Design review of the part built by this model. Coordinates are the model's own, in mm. Face numbers are marked on the shaded views. Round coordinates to 2 decimals unless told otherwise and drop trailing zeros. Write each loop counter-clockwise with the first axis right and the second up, starting at its lowest first coordinate (ties: lowest second). Pieces come first, ordered by that corner, then holes. Notation, with made-up numbers: M -7,-6 L 49,-6 A18 ccw 49,10 Z; hole C 31.5,2 d10. An arc over 180 degrees is marked long. One line per question, with ' | ' between items. Start each with the question number.
Item 1: Insertion check: pin 1 Ø1.5 at (x, z) = (4.5, 2.5) entering from -Y; pin 2 Ø1 at (y, z) = (9, -3.5) entering from -X; pin 3 Ø4 at (x, y) = (-4, 5) entering from -Z; pin 4 Ø5 at (y, z) = (9, -3.5) entering from +X. Each pin has a flat end and moves straight along its axis. Give the tip position at first contact, or say it passes through.
Item 2: Add section A-A, the plane x = 0. State the section outline as (y, z) points.
Item 3: Add section C-C, the plane y = 1.75. State the section outline as (x, z) points.
Item 4: Draft analysis for pull direction Z (two halves, no side actions). For the marked faces 1, 2 and 3, state which applies: released by +Z, released by -Z, zero draft, split by the parting line, or undercut.
Item 5: Add section B-B, the plane z = 0. State the section outline as (x, y) points, and give its area (3 significant figures).
Item 6: For L1, parallel to Z at x = 0, y = 6; L2, parallel to X at y = 3.25, z = -2; L3, parallel to Z at x = 2.25, y = 4.5, list the stretches that pass through material, from the lowest coordinate up.
```python
from build123d import *

# Parameters (mm, degrees)
F0_R     = 6.5
F0_R_2   = 4
F1_DEPTH = 12
F2_SIZE  = 0.3


with BuildPart() as f1:
    # F0 (on Front) → F1 (new body)
    with BuildSketch(Plane.XZ):
        Circle(F0_R)
        Circle(F0_R_2, mode=Mode.SUBTRACT)
    extrude(amount=-F1_DEPTH)

    # F2
    f2_edges = [f1.edges().sort_by_distance(p)[0] for p in [
        (-6.5, 0, 0),
        (-6.5, 12, 0),
        (-4, 0, 0),
        (-4, 12, 0),
    ]]
    chamfer(f2_edges, length=F2_SIZE)


solid = f1.part
```
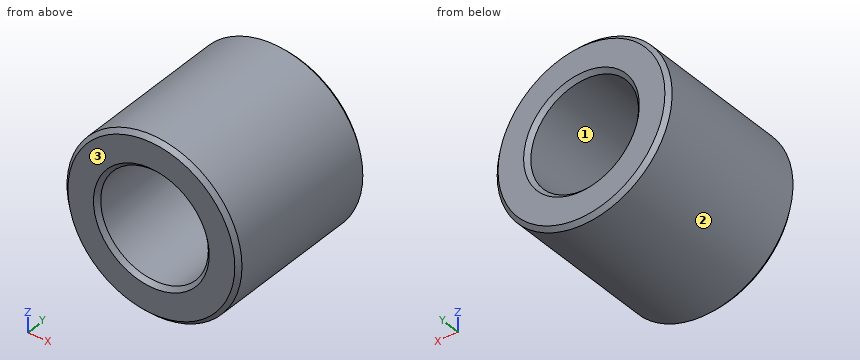
Computed values:
1) pin 1: stops at y = 0 | pin 2: stops at x = -5.77 | pin 3: stops at z = -6.18 | pin 4: stops at x = 6.42
2) outline: M 0,-6.2 L 0.3,-6.5 L 11.7,-6.5 L 12,-6.2 L 12,-4.3 L 11.7,-4 L 0.3,-4 L 0,-4.3 Z; M 0,4.3 L 0.3,4 L 11.7,4 L 12,4.3 L 12,6.2 L 11.7,6.5 L 0.3,6.5 L 0,6.2 Z
3) outline: C 0,0 d13; hole C 0,0 d8
4) face 1: undercut | face 2: split by the parting line | face 3: zero draft
5) outline: M -6.5,0.3 L -6.2,0 L -4.3,0 L -4,0.3 L -4,11.7 L -4.3,12 L -6.2,12 L -6.5,11.7 Z; M 4,0.3 L 4.3,0 L 6.2,0 L 6.5,0.3 L 6.5,11.7 L 6.2,12 L 4.3,12 L 4,11.7 Z | area: 59.6 mm^2
6) L1: z = -6.5 to -4, 4 to 6.5 | L2: x = -6.18 to -3.46, 3.46 to 6.18 | L3: z = -6.1 to -3.31, 3.31 to 6.1
